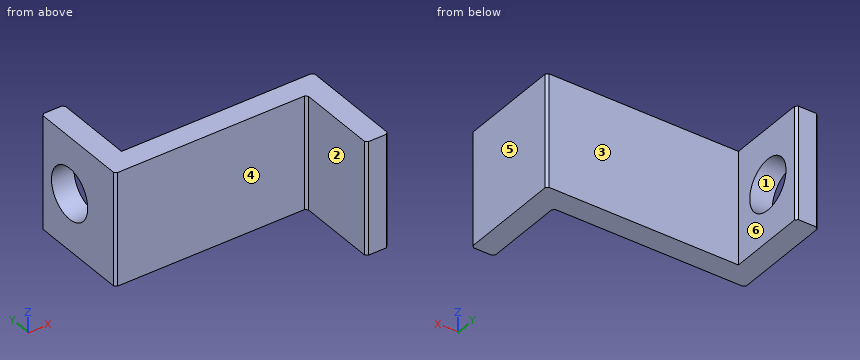
```python
from build123d import *

# Parameters (mm, degrees)
BOSS_EXTRU_1_DEPTH = 10
CHANFREIN2_SIZE    = 0.2
D_GAGEMENT_M41_D   = 4.5


with BuildPart() as part:
    # Esquisse1 → Boss.-Extru.1 (new body)
    with BuildSketch(Plane.XY):
        Polygon((0, 32), (0, 41.35), (-17, 41.35), (-17, 48.5), (-19, 48.5), (-19, 39.35), (-2, 39.35), (-2, 32), align=None)
    extrude(amount=BOSS_EXTRU_1_DEPTH)

    # Chanfrein2
    chanfrein2_edges = [part.edges().sort_by_distance(p)[0] for p in [
        (0, 41.35, 5),
        (0, 32, 5),
        (-2, 32, 5),
        (-2, 39.35, 5),
        (-19, 39.35, 5),
        (-19, 48.5, 5),
        (-17, 48.5, 5),
    ]]
    chamfer(chanfrein2_edges, length=CHANFREIN2_SIZE)

    # Dégagement M41 (through all)
    with Locations(Plane.ZY.offset(19)):
        with Locations((5, 45)):
            Hole(D_GAGEMENT_M41_D / 2)


solid = part.part
```
Here's how the part is built. I have some questions about the finished solid (model axes, mm). Face numbers are marked on the shaded views. A direction names the side the tool comes from. Give positions to 0.01 mm unless a question says otherwise; leave off trailing zeros. Write each loop counter-clockwise with the first axis right and the second up, starting at its lowest first coordinate (ties: lowest second). Pieces come first, ordered by that corner, then holes.
(1) Imagine slicing it at D-D, the plane y = 42. Write out the boundary of the cut face in (x, z), and give its area (3 significant figures).
Output values:
outline: (-19, 0) - (-17, 0) - (-17, 10) - (-19, 10) - close
area: 20.0 mm2
(2) Will these pins go through, and if not, where does the flat tip stop? pin 1 (6 mm diameter, centred on y = 33.5, z = 1.5, fed in from -X); pin 2 (5.5 mm diameter, centred on y = 46.5, z = 4, fed in from +X).
Output values:
pin 1: stops at x = -2
pin 2: stops at x = -17
(3) Imagine slicing it at A-A, the plane y = 45. Write out the boundary of the cut face in (x, z), and give its area (3 significant figures).
Output values:
outline: (-19, 0) - (-17, 0) - (-17, 2.75) - (-19, 2.75) - close; (-19, 7.25) - (-17, 7.25) - (-17, 10) - (-19, 10) - close
area: 11.0 mm2
(4) Thinking about a two-plate mould opening in Y: for the marked faces 1, 2 and 3, which applies, pulls with the +Y half, pulls with the -Y half, needs draft (parallel to the pull), parting line crosses it, or undercut?
Output values:
face 1: undercut
face 2: needs draft
face 3: pulls with the +Y half
(5) On a 3-axis mill with a long thin cutter (end or side, diameter ignored), from which of +Z, -Z, +X, -X, +Y, -Y can I reach the whole of each face in a straight line? I mean the marked faces 4, 5 and 6. Say none if no direction works.
Output values:
face 4: +Z, -Z, -X, -Y
face 5: +Z, -Z, +X, +Y, -Y
face 6: +Z, -Z, +X, +Y
(6) Imagine slicing it at C-C, the plane z = 7.5. Write out the boundary of the cut face in (x, y).
Output values:
outline: (-19, 39.55) - (-18.8, 39.35) - (-2.2, 39.35) - (-2, 39.15) - (-2, 32.2) - (-1.8, 32) - (-0.2, 32) - (0, 32.2) - (0, 41.15) - (-0.2, 41.35) - (-17, 41.35) - (-17, 48.3) - (-17.2, 48.5) - (-18.8, 48.5) - (-19, 48.3) - close
(7) Imagine slicing it at B-B, the plane z = 5. Write out the boundary of the cut face in (x, y), and give its area (3 significant figures).
Output values:
outline: (-19, 39.55) - (-18.8, 39.35) - (-2.2, 39.35) - (-2, 39.15) - (-2, 32.2) - (-1.8, 32) - (-0.2, 32) - (0, 32.2) - (0, 41.15) - (-0.2, 41.35) - (-17, 41.35) - (-17, 42.75) - (-19, 42.75) - close; (-19, 47.25) - (-17, 47.25) - (-17, 48.3) - (-17.2, 48.5) - (-18.8, 48.5) - (-19, 48.3) - close
area: 57.9 mm2
(8) If I drill on L1, parallel to Y at x = -18, z = 5; L2, parallel to X at y = 36, z = 7.75; L3, parallel to Y at x = -7.25, z = 4, over which ranges is the centre line in solid material (lowest first)?
Output values:
L1: y = 39.35 to 42.75, 47.25 to 48.5
L2: x = -2 to 0
L3: y = 39.35 to 41.35
